Autodesk Inventor part; units mm, degrees
ref_plane "YZ Plane" through (0, 0, 0) normal (1, 0, 0) x (0, 1, 0)
ref_plane "XY Plane" through (0, 0, 0) normal (0, 0, 1) x (1, 0, 0)
sketch "Sketch4" plane through (0, 0, 0) normal (1, 0, 0) x (0, 1, 0)
  line L0 (-25.4, 15.875) -> (-25.4, -15.875)
  line L1 (-25.4, -15.875) -> (25.4, -15.875)
  line L2 (25.4, -15.875) -> (25.4, 15.875)
  line L3 (25.4, 15.875) -> (-25.4, 15.875)
  line L4 (-25.4, 15.875) -> (25.4, -15.875) construction
  line L5 (-25.4, -15.875) -> (25.4, 15.875) construction
  point P0 (0, 0)
  dimension "d11" = 50.8
  dimension "d12" = 31.75
extrude "Extrusion4" add sketch "Sketch4" along normal blind 6.35
sketch "Sketch5" plane through (0, 0, 0) normal (-1, 0, 0) x (0, 0, 1)
  circle A0 centre (0, 0) radius 2.6543
  dimension "d15" = 5.3086
extrude "Extrusion5" cut sketch "Sketch5" against normal through all
sketch "Sketch7" plane through (6.35, 0, 0) normal (1, 0, 0) x (0, 0, -1)
  line L0 (15.875, 25.4) -> (-15.875, 25.4)
  line L1 (-9.525, 25.4) -> (9.525, 25.4)
  line L2 (9.525, 25.4) -> (9.525, 21.717)
  line L3 (9.525, 21.717) -> (-9.525, 21.717)
  line L4 (-9.525, 21.717) -> (-9.525, 25.4)
  line L5 (-15.875, 25.4) -> (-15.875, -25.4)
  point P0 (0, 0)
  dimension "d25" = 19.05
  dimension "d26" = 6.35
  dimension "d27" = 3.683
extrude "Extrusion7" cut sketch "Sketch7" against normal through all
mirror "Mirror2" about plane through (0, 0, 0) normal (0, 1, 0) of "Extrusion7"
sketch "Sketch8" plane through (6.35, 0, 0) normal (1, 0, 0) x (0, 0, -1)
  line L0 (0, 12.192) -> (7.62, 12.192)
  line L1 (7.62, 12.192) -> (7.62, 21.717)
  line L2 (7.62, 21.717) -> (-7.62, 21.717)
  line L3 (-7.62, 21.717) -> (-7.62, 12.192)
  line L4 (-7.62, 12.192) -> (0, 12.192)
  line L5 (9.525, 21.717) -> (-9.525, 21.717)
  point P0 (0, 0)
  dimension "d30" = 9.525
  dimension "d32" = 7.62
  dimension "d33" = 7.62
extrude "Extrusion8" cut sketch "Sketch8" against normal through all
mirror "Mirror3" about plane through (0, 0, 0) normal (0, 1, 0) of "Extrusion8"
equation "\"d11\" = pushPlateLength"
equation "\"d12\" = pushPlateWidth"
equation "\"stopMechanismWidth\" = 50.8"
equation "\"materialThickness\" = 3.175"
equation "\"stopMechanismLength\" = 50.8"
equation "\"stopMEchamismHeight\" = 50.8"
equation "\"stopMechanismHoleForPost\" = 9.525"
equation "\"pushPlateLength\" = 50.8"
equation "\"pushPlateWidth\" = 31.75"
equation "\"slotWidth\" = 12.7"
equation "\"slotDepth\" = 9.525"
properties part number "StopMechanismPushPlate" material "Aluminum 6061"
Can you work these out from the model? Positions are in its coordinate system, mm. A direction names the side the tool comes from. Round coordinates to 2 decimals unless told otherwise and drop trailing zeros. Loops run counter-clockwise (first coordinate to the right, second up) from the corner with the lowest first, then second, coordinate; pieces in that order, holes last. Notation, with made-up numbers: M 39,-1 L 50,-1 A22 cw 50,7 Z; hole C 72,-8.75 d10. An arc over 180 degrees is marked long. Write item = value, one per line. Start each with the question number.
(1) Suppose I cut it at D-D on z = -4. Write out the boundary of the cut face in (x, y).
(2) If we mould it in two halves opening along Y, with no side actions, what happens to faces 1 (the face through (3.13, 0.8, 2.53)), 2 (the face through (3, 12.192, 0)), 3 (the face through (0, 0, 4))? For each: released by +Y, released by -Y, zero draft, split by the parting line, or undercut.
(3) I'm going to push flat-ended pins straight in: P1, Ø5, axis at y = 16, z = -0.5, coming from the +X side; P2, Ø2, axis at x = 5.5, z = 1.5, coming from the +Y side; P3, Ø0.6, axis at x = 4.5, z = 8.5, coming from the +Y side; P4, Ø1.9, axis at x = 4.5, z = 3.5, coming from the -Y side. Where does each tip first touch, or does it pass through?
(4) Which directions (+Z, -Z, +X, -X, +Y, -Y) give clear straight access to the entire face, cutting with the end or side of a thin tool? Please do faces 4 (the face through (3, 0, -15.875)), 5 (the face through (3, 24, 9.525)), 6 (the face through (3, -24, -9.525)).
(5) Suppose I cut it at A-A on z = 0. Write out the boundary of the cut face in (x, y).
(6) I need wall thicknesses on line 1 along Y through (x, z) = (1.5, 0); line 2 along Z through (x, y) = (5.75, 17) (3 decimals); line 3 along Y through (x, z) = (3, 5). Which ranges of each line are inside material? Lowest first, please.
(7) Suppose I cut it at C-C on x = 2.75. Write out the boundary of the cut face in (y, z) (3 decimals), plus the area to 3 significant figures.
(8) Suppose I cut it at B-B on y = 0. Write out the boundary of the cut face in (x, z) (3 decimals), plus the area to 3 significant figures.
Answer block:
q1.outline = M 0,-12.19 L 6.35,-12.19 L 6.35,12.19 L 0,12.19 Z
q2.face_1 = undercut
q2.face_2 = released by +Y
q2.face_3 = zero draft
q3.P1 = through
q3.P2 = 12.19
q3.P3 = 21.72
q3.P4 = -12.19
q4.face_4 = -Z, +X, -X, +Y, -Y
q4.face_5 = +X, -X, +Y
q4.face_6 = +X, -X, -Y
q5.outline = M 0,-12.19 L 6.35,-12.19 L 6.35,-2.65 L 0,-2.65 Z; M 0,2.65 L 6.35,2.65 L 6.35,12.19 L 0,12.19 Z
q6.line_1 = -12.19 to -2.65, 2.65 to 12.19
q6.line_2 = -15.875 to -7.62, 7.62 to 15.875
q6.line_3 = -12.19 to 12.19
q7.outline = M -25.4,-15.875 L 25.4,-15.875 L 25.4,-9.525 L 21.717,-9.525 L 21.717,-7.62 L 12.192,-7.62 L 12.192,7.62 L 21.717,7.62 L 21.717,9.525 L 25.4,9.525 L 25.4,15.875 L -25.4,15.875 L -25.4,9.525 L -21.717,9.525 L -21.717,7.62 L -12.192,7.62 L -12.192,-7.62 L -21.717,-7.62 L -21.717,-9.525 L -25.4,-9.525 Z; hole C 0,0 d5.309
q7.area = 1,160 mm²
q8.outline = M 0,-15.875 L 6.35,-15.875 L 6.35,-2.654 L 0,-2.654 Z; M 0,2.654 L 6.35,2.654 L 6.35,15.875 L 0,15.875 Z
q8.area = 168 mm²
